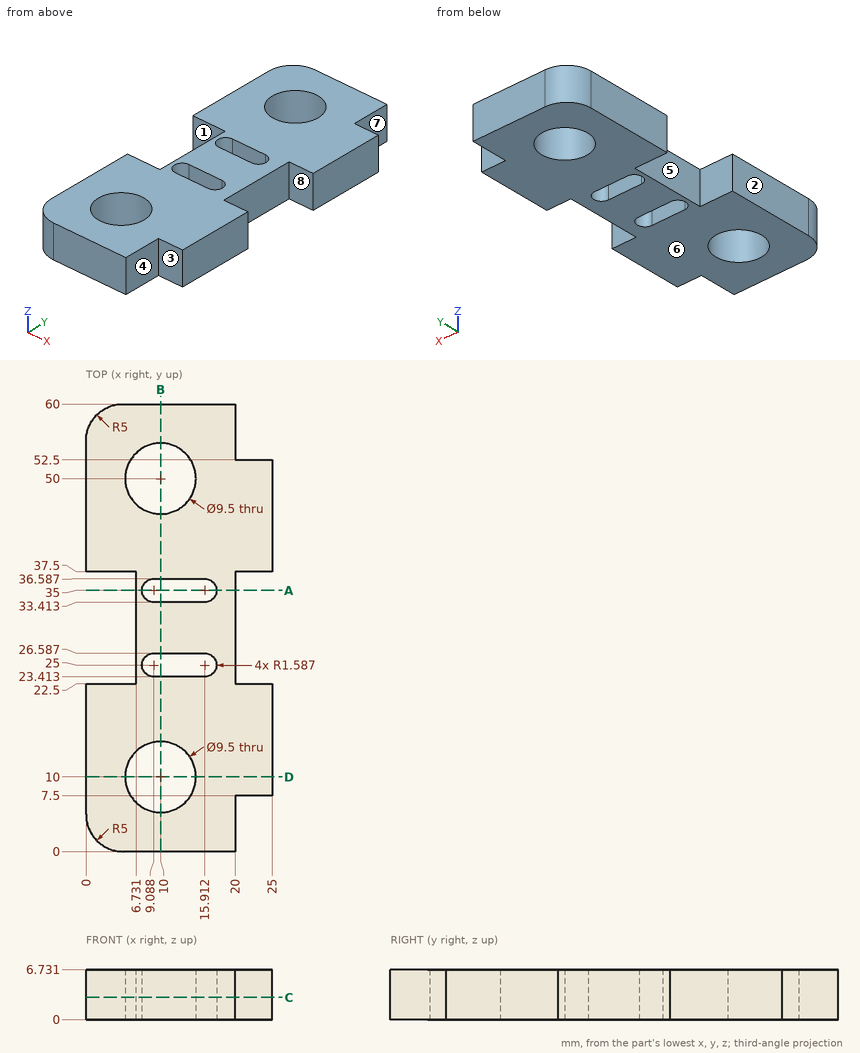
For this review, use the dimensioned drawing (mm, ordinates from the lowest corner) and the shaded views. A direction names the side the tool comes from. Round coordinates to 2 decimals unless told otherwise and drop trailing zeros. Order: outer loops, then holes, each group sorted by start corner. A loop starts at its lowest first (then second) coordinate and runs counter-clockwise, first axis right, second up.
1) Draft analysis for pull direction Y (two halves, no side actions). For the marked faces 1, 2 and 3, state which applies: released by +Y, released by -Y, zero draft, split by the parting line, or undercut.
The answers:
face 1: undercut
face 2: zero draft
face 3: released by -Y
2) Machinability: for the marked faces 4, 5, 6, 7 and 8, which of the approach directions +Z, -Z, +X, -X, +Y, -Y give a long, thin tool a straight path to every point of the face, cutting with its end or side? Answer none if there is none.
The answers:
face 4: +Z, -Z, +X, -Y
face 5: +Z, -Z, -X
face 6: -Z, +X, -X, +Y, -Y
face 7: +Z, -Z, +X, +Y
face 8: +Z, -Z, +X
3) Consider section D-D (y = 10). State the section outline as (x, z) points, plus the area to 3 significant figures.
The answers:
outline: (0, 0) - (5.25, 0) - (5.25, 6.73) - (0, 6.73) - close; (14.75, 0) - (25, 0) - (25, 6.73) - (14.75, 6.73) - close
area: 104 mm2
4) For L1, parallel to Y at x = 10, z = 5; L2, parallel to Y at x = 23.25, z = 5.25; L3, parallel to Y at x = 7.75, z = 4.5 (1 decimal), list the stretches that pass through material, from the lowest coordinate up.
The answers:
L1: y = 0 to 5.25, 14.75 to 23.41, 26.59 to 33.41, 36.59 to 45.25, 54.75 to 60
L2: y = 7.5 to 22.5, 37.5 to 52.5
L3: y = 0 to 5.8, 14.2 to 24.1, 25.9 to 34.1, 35.9 to 45.8, 54.2 to 60
5) Consider section C-C (z = 3). Count the separate pieces of the cut face and the enclosed holes in it, plus the area to 3 significant figures.
The answers:
separate pieces: 1
enclosed holes: 4
area: 1,040 mm2
6) Consider section B-B (x = 10). State the section outline as (y, z) points, plus the area to 3 significant figures.
The answers:
outline: (0, 0) - (5.25, 0) - (5.25, 6.73) - (0, 6.73) - close; (14.75, 0) - (23.41, 0) - (23.41, 6.73) - (14.75, 6.73) - close; (26.59, 0) - (33.41, 0) - (33.41, 6.73) - (26.59, 6.73) - close; (36.59, 0) - (45.25, 0) - (45.25, 6.73) - (36.59, 6.73) - close; (54.75, 0) - (60, 0) - (60, 6.73) - (54.75, 6.73) - close
area: 233 mm2
7) Clearance check with flat-ended pins moving along their axes: pin 1 Ø3.5 at (y, z) = (27.5, 3.5) entering from -X; pin 2 Ø12 at (x, y) = (15, 21) entering from -Z; pin 3 Ø4 at (x, z) = (22.5, 3.5) entering from -Y; pin 4 Ø2 at (y, z) = (57, 4) entering from +X. State where each tip first meets the part, or that it passes through.
The answers:
pin 1: stops at x = 6.73
pin 2: stops at z = 0
pin 3: stops at y = 7.5
pin 4: stops at x = 20
8) Consider section A-A (y = 35). State the section outline as (x, z) points.
The answers:
outline: (6.73, 0) - (7.5, 0) - (7.5, 6.73) - (6.73, 6.73) - close; (17.5, 0) - (20, 0) - (20, 6.73) - (17.5, 6.73) - close
